from build123d import *

# Parameters (mm, degrees)
F0_R        = 2
F1_DEPTH    = 10
F2_DEPTH    = 5.25
F3_T1_DEPTH = 44.4948974279


# Not quite as in the source:
# - a fillet or chamfer that OpenCascade refuses, or shapes differently, is made with other operations: its cross-section is extruded or revolved along the edge and cut away or added


with BuildPart() as f1:
    # F0 (on Top) → F1 (new body, symmetric)
    with BuildSketch(Plane.XY):
        with BuildLine():
            Line((64, 0), (0, 0))
            Line((0, 0), (0, -4))
            Line((0, -4), (60, -4))
            ThreePointArc((60, -4), (61.1715728753, -1.1715728753), (64, 0))
        make_face()
        with BuildLine():
            ThreePointArc((68, -4), (66.8284271247, -1.1715728753), (64, 0))
            ThreePointArc((64, 0), (61.1715728753, -1.1715728753), (60, -4))
            ThreePointArc((60, -4), (64, -8), (68, -4))
        make_face()
        with Locations((64, -4)):
            Circle(F0_R, mode=Mode.SUBTRACT)
    extrude(amount=F1_DEPTH, both=True)

    # F0 (on Top) → F2 (cut, symmetric)
    with BuildSketch(Plane.XY):
        with BuildLine():
            ThreePointArc((68, -4), (66.8284271247, -1.1715728753), (64, 0))
            ThreePointArc((64, 0), (61.1715728753, -1.1715728753), (60, -4))
            ThreePointArc((60, -4), (64, -8), (68, -4))
        make_face()
        with Locations((64, -4)):
            Circle(F0_R, mode=Mode.SUBTRACT)
    extrude(amount=F2_DEPTH, both=True, mode=Mode.SUBTRACT)

    # F3: fillet of radius 5 on 1 edges, made by hand

    # F3_s2 → F3_t1 (cut)
    with BuildSketch(Plane.XY.offset(-22.2474487139)):
        with BuildLine():
            ThreePointArc((4.8989794856, -4), (1.7367018254, -2.8729833462), (0, 0))
            Line((0, 0), (0, -4))
            Line((0, -4), (4.8989794856, -4))
        make_face()
    extrude(amount=F3_T1_DEPTH, mode=Mode.SUBTRACT)


solid = f1.part
The listing builds one solid part. Answer for the finished solid, in the listing's coordinates (mm). A direction names the side the tool comes from. Give positions to 0.01 mm unless a question says otherwise; leave off trailing zeros. Write each loop counter-clockwise with the first axis right and the second up, starting at its lowest first coordinate (ties: lowest second). Pieces come first, ordered by that corner, then holes. Notation, with made-up numbers: (29.5, 24.5) - (42.5, 24.5) arc R3 cw to (42.5, 29.5) - close; hole circle Ø4 at (61, 40). An arc over 180 degrees is marked (long way). Use a Markdown table: item, result.
1. Each of these flat-tipped pins is pushed along its axis until it touches: P1, Ø10, axis at x = 44, z = 1, coming from the -Y side; P2, Ø1.5, axis at y = -1, z = -3, coming from the -X side. Where does it stop, or does it pass through?
Values follow:
| item | result |
|---|---|
| P1 | stops at y = -4 |
| P2 | stops at x = 0.06 |
2. Section C-C on y = -1 is taken. Write down the section's boundary in (x, z), plus the area to 3 significant figures.
Values follow:
| item | result |
|---|---|
| outline | (0.32, -10) - (66.65, -10) - (66.65, -5.25) - (61.35, -5.25) - (61.35, 5.25) - (66.65, 5.25) - (66.65, 10) - (0.32, 10) - close |
| area | 1,270 mm² |
3. Section B-B on z = 8.5 is taken. Write down the section's boundary in (x, y), plus the area to 3 significant figures.
Values follow:
| item | result |
|---|---|
| outline | (0, 0) arc R5 ccw to (4.9, -4) - (60, -4) arc R4 ccw (long way) to (64, 0) - close; hole circle Ø4 at (64, -4) |
| area | 276 mm² |
4. Section D-D on x = 55 is taken. Write down the section's boundary in (y, z).
Values follow:
| item | result |
|---|---|
| outline | (-4, -10) - (0, -10) - (0, 10) - (-4, 10) - close |
5. Find the intervals of material crossed by probe 1 along Y at (x, z) = (64, 7.25); probe 2 along Y at (x, z) = (56, 1.75); probe 3 along Z at (x, y) = (64, -1.5), in increasing order. Write a range as from..to.
Values follow:
| item | result |
|---|---|
| probe 1 | y = -8..-6, -2..0 |
| probe 2 | y = -4..0 |
| probe 3 | z = -10..-5.25, 5.25..10 |
6. For a pull along Y with two mould halves and no side action, classify faces 1 (the cylindrical face through (62, -4, 8)), 2 (the cylindrical face through (1.77, -2.9, -0.14)), 3 (the flat face through (62, -5, -5.25)) as released by +Y, released by -Y, zero draft, split by the parting line, or undercut.
Values follow:
| item | result |
|---|---|
| face 1 | undercut |
| face 2 | released by -Y |
| face 3 | zero draft |
7. Section A-A on y = -5 is taken. Write down the section's boundary in (x, z).
Values follow:
| item | result |
|---|---|
| outline | (60.13, -10) - (62.27, -10) - (62.27, -5.25) - (60.13, -5.25) - close; (60.13, 5.25) - (62.27, 5.25) - (62.27, 10) - (60.13, 10) - close; (65.73, -10) - (67.87, -10) - (67.87, -5.25) - (65.73, -5.25) - close; (65.73, 5.25) - (67.87, 5.25) - (67.87, 10) - (65.73, 10) - close |
8. A tool of negligible diameter and unlimited length cuts with its end or side. For faces 4 (the flat face through (32, 0, 0)), 5 (the cylindrical face through (61.203, -1.141, 0.074)), 6 (the flat face through (32, -4, 0)), from which of +Z, -Z, +X, -X, +Y, -Y can it reach the whole face along a straight path? Write none if from no direction.
Values follow:
| item | result |
|---|---|
| face 4 | +Z, -Z, +X, -X, +Y |
| face 5 | +X, -Y |
| face 6 | +Z, -Z, -X, -Y |
